```python
from build123d import *

# Parameters (mm, degrees)
F0_R     = 3.37213
F0_R_2   = 2.330993
F0_R_3   = 3.361663
F1_DEPTH = 2


with BuildPart() as f1:
    # F0 (on Top) → F1 (new body)
    with BuildSketch(Plane.XY):
        with BuildLine():
            ThreePointArc((3.313187, 14.629518), (-0.627308, 20.006438), (-4.223204, 14.393212))
            ThreePointArc((-4.223204, 14.393212), (0.470099, -14.992632), (3.313187, 14.629518))
        make_face()
        with BuildLine():
            ThreePointArc((9.486387, -2.59901), (-0.12995, -9.889774), (-9.746287, -2.59901))
            ThreePointArc((-9.746287, -2.59901), (-0.12995, -5.751122), (9.486387, -2.59901))
        make_face(mode=Mode.SUBTRACT)
        with Locations((-5.515314, 6.171075)):
            Circle(F0_R, mode=Mode.SUBTRACT)
        with Locations((-0.500647, 15.966899)):
            Circle(F0_R_2, mode=Mode.SUBTRACT)
        with Locations((2.455175, 6.630911)):
            Circle(F0_R_3, mode=Mode.SUBTRACT)
    extrude(amount=F1_DEPTH)


solid = f1.part
```
Source: CAD feature listing. Evaluate the final solid. Frame: model axes, mm. Give positions to 0.01 mm unless a question says otherwise; leave off trailing zeros. Write each loop counter-clockwise with the first axis right and the second up, starting at its lowest first coordinate (ties: lowest second). Pieces come first, ordered by that corner, then holes.
1. Section query C-C (y = -4.5). Return the cut outline in (x, z).
2. Section query B-B (x = 6.5). Return the cut outline in (y, z), then the cut area to 3 significant figures.
3. Pull-direction query (X, two-part tool) for faces 1 (the face through (-2.4, 4.88, 0.99)), 2 (the face through (0, 3, 0)), 3 (the face through (0, -15, 1)); classes: +X half, -X half, draft (parallel to the pull), parting line (faces both ways), or undercut.
4. Section query A-A (x = -0.5). Return the cut outline in (y, z), then the cut area to 3 significant figures.
5. Section query D-D (z = 1). Return the cut outline in (x, y).
6. Material intervals for line 1 along X through (y, z) = (16, 0.65); line 2 along Y through (x, z) = (5.5, 0.25); line 3 along Y through (x, z) = (3, 1.95), sorted ascending.
Output values:
1. outline: (-14.31, 0) - (-9, 0) - (-9, 2) - (-14.31, 2) - close; (-6.38, 0) - (6.12, 0) - (6.12, 2) - (-6.38, 2) - close; (8.74, 0) - (14.31, 0) - (14.31, 2) - (8.74, 2) - close
2. outline: (-13.52, 0) - (-7.37, 0) - (-7.37, 2) - (-13.52, 2) - close; (-4.34, 0) - (13.52, 0) - (13.52, 2) - (-4.34, 2) - close
2. area: 48.0 mm2
3. face 1: undercut
3. face 2: draft
3. face 3: parting line
4. outline: (-14.99, 0) - (-9.88, 0) - (-9.88, 2) - (-14.99, 2) - close; (-5.75, 0) - (5.03, 0) - (5.03, 2) - (-5.75, 2) - close; (8.23, 0) - (13.64, 0) - (13.64, 2) - (8.23, 2) - close; (18.3, 0) - (20.01, 0) - (20.01, 2) - (18.3, 2) - close
4. area: 46.0 mm2
5. outline: (-4.22, 14.39) arc R15 ccw (long way) to (3.31, 14.63) arc R4.04 ccw (long way) to start; hole (-9.75, -2.6) arc R9.99 ccw to (9.49, -2.6) arc R16.24 cw to start; hole circle Ø6.74 at (-5.52, 6.17); hole circle Ø4.66 at (-0.5, 15.97); hole circle Ø6.72 at (2.46, 6.63)
6. line 1: x = -4.54 to -2.83, 1.83 to 3.54
6. line 2: y = -13.96 to -8.15, -4.74 to 5.21, 8.06 to 13.96
6. line 3: y = -14.7 to -9.39, -5.45 to 3.31, 9.95 to 17.99
